Geometry check sheet. Reference: drawing and pictorial views, mm from the part's lowest x, y, z. A direction names the side the tool comes from. Give positions to 0.01 mm unless a question says otherwise; leave off trailing zeros. Loops run counter-clockwise (first coordinate to the right, second up) from the corner with the lowest first, then second, coordinate; pieces in that order, holes last. Notation, with made-up numbers: (-7, -36) - (25, -36) arc R8 ccw to (25, -24) - close; hole circle Ø8 at (87, -37). An arc over 180 degrees is marked (long way). Use CSV: the item, a comma, the result in double quotes.
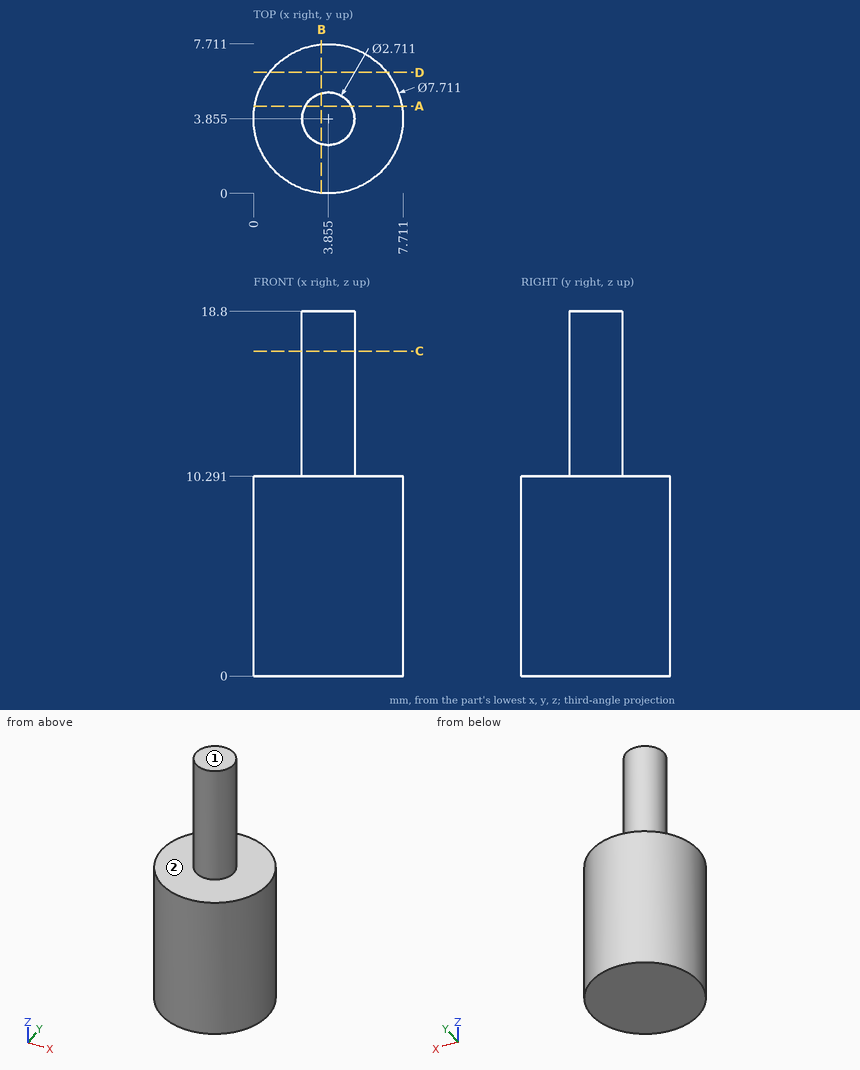
1. Sectioned sample at C-C, the plane z = 16.75. Record the boundary of the cut face in (x, y) (1 decimal).
Completed:
outline,"circle Ø2.7 at (3.9, 3.9)"
2. Sectioned sample at A-A, the plane y = 4.5. Record the boundary of the cut face in (x, z) (1 decimal).
Completed:
outline,"(0.1, 0) - (7.7, 0) - (7.7, 10.3) - (5, 10.3) - (5, 18.8) - (2.7, 18.8) - (2.7, 10.3) - (0.1, 10.3) - close"
3. Sectioned sample at B-B, the plane x = 3.5. Record the boundary of the cut face in (y, z) (1 decimal), and give its area (3 significant figures).
Completed:
outline,"(0, 0) - (7.7, 0) - (7.7, 10.3) - (5.2, 10.3) - (5.2, 18.8) - (2.5, 18.8) - (2.5, 10.3) - (0, 10.3) - close"
area,"101 mm²"
4. Sectioned sample at D-D, the plane y = 6.25. Record the boundary of the cut face in (x, z).
Completed:
outline,"(0.83, 0) - (6.88, 0) - (6.88, 10.29) - (0.83, 10.29) - close"
5. Go/stop test with flat-tipped pins: pin 1 Ø2 at (x, y) = (3, 5) entering from -Z; pin 2 Ø2 at (x, z) = (1.5, 6) entering from +Y (1 decimal). Record where each tip stops, or that it passes through.
Completed:
pin 1,"stops at z = 0"
pin 2,"stops at y = 7.5"
6. Set-up check for the marked faces 1 and 2: record each of +Z, -Z, +X, -X, +Y, -Y from which the full face is reachable in a straight line by a thin tool's end or side.
Completed:
face 1,"+Z, +X, -X, +Y, -Y"
face 2,"+Z"
7. Scan lines: line 1 along Z through (x, y) = (6, 3.5); line 2 along Y through (x, z) = (2, 9.5) (1 decimal); line 3 along X through (y, z) = (6.25, 8.75) (1 decimal). Record each from-to range of solid material in increasing order.
Completed:
line 1,"z = 0 to 10.29"
line 2,"y = 0.5 to 7.2"
line 3,"x = 0.8 to 6.9"
